Geometry check sheet. Reference: drawing and pictorial views, mm from the part's lowest x, y, z. Give positions to 0.01 mm unless a question says otherwise; leave off trailing zeros. Loops run counter-clockwise (first coordinate to the right, second up) from the corner with the lowest first, then second, coordinate; pieces in that order, holes last. Notation, with made-up numbers: (87, 42) - (110, 42) arc R14 ccw to (110, 60) - close; hole circle Ø10 at (19, 16.25). An arc over 180 degrees is marked (long way). Answer in a Markdown table with one row per item. Add a question column.
(1) Sectioned sample at D-D on z = 4.5. Enter the section's corners in (x, y), then the cut area to 3 significant figures.
(2) Sectioned sample at C-C on y = 15. Enter the section's corners in (x, z).
(3) Thickness scan on L1, parallel to X at y = 1.75, z = 5; L2, parallel to Z at x = 8, y = 17; L3, parallel to X at y = 7.75, z = 4.25. Record the ranges inside material, lowest first.
(4) Go/stop test with a flat-tipped pin: P1, Ø3, axis at x = 32, z = 6.5, coming from the -Y side. Record where the tip stops, or that it passes through.
(5) Sectioned sample at A-A on z = 6.5. Enter the section's corners in (x, y).
(6) Draft check along Z on the marked faces 1, 2, 3 and 4. Enter one of: released by +Z, released by -Z, zero draft, split by the parting line, or undercut.
(7) Sectioned sample at B-B on x = 32. Enter the section's corners in (y, z), then the cut area to 3 significant figures.
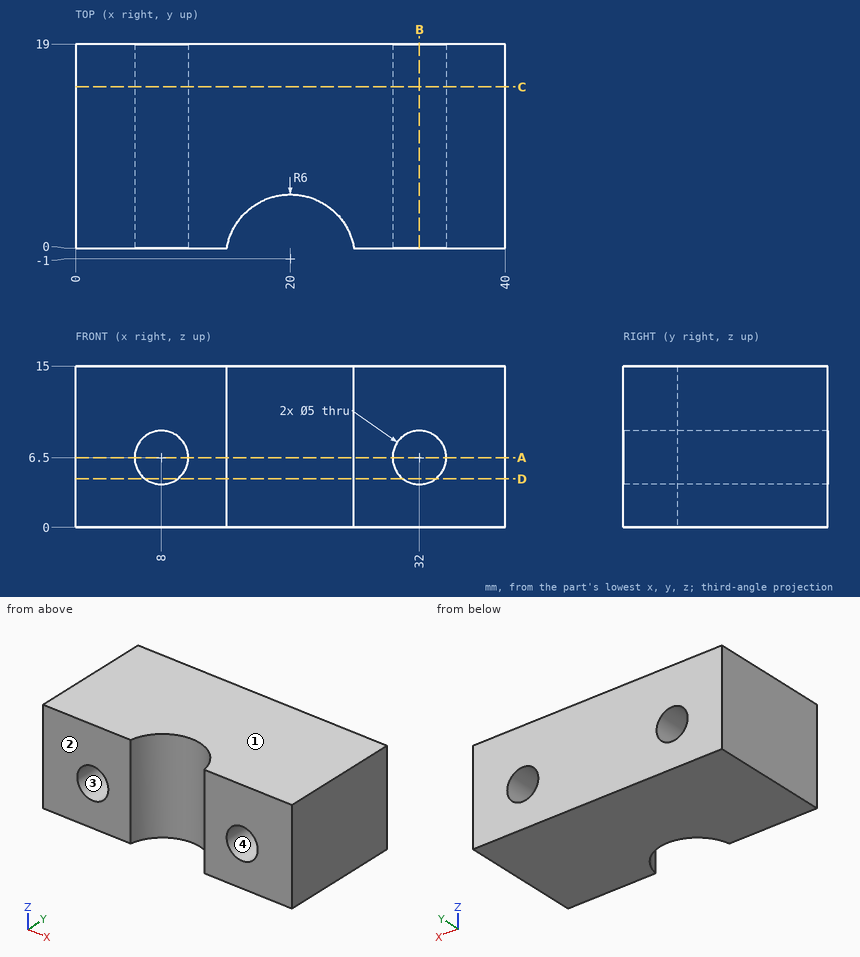
Reply:
| question | item | result |
|---|---|---|
| 1 | outline | (0, 0) - (6.5, 0) - (6.5, 19) - (0, 19) - close; (9.5, 0) - (14.08, 0) arc R6 cw to (25.92, 0) - (30.5, 0) - (30.5, 19) - (9.5, 19) - close; (33.5, 0) - (40, 0) - (40, 19) - (33.5, 19) - close |
| 1 | area | 601 mm^2 |
| 2 | outline | (0, 0) - (40, 0) - (40, 15) - (0, 15) - close; hole circle Ø5 at (8, 6.5); hole circle Ø5 at (32, 6.5) |
| 3 | L1 | 0 to 6, 10 to 14.67, 25.33 to 30, 34 to 40 |
| 3 | L2 | 0 to 4, 9 to 15 |
| 3 | L3 | 0 to 6.91, 9.09 to 30.91, 33.09 to 40 |
| 4 | P1 | through |
| 5 | outline | (0, 0) - (5.5, 0) - (5.5, 19) - (0, 19) - close; (10.5, 0) - (14.08, 0) arc R6 cw to (25.92, 0) - (29.5, 0) - (29.5, 19) - (10.5, 19) - close; (34.5, 0) - (40, 0) - (40, 19) - (34.5, 19) - close |
| 6 | face 1 | released by +Z |
| 6 | face 2 | zero draft |
| 6 | face 3 | undercut |
| 6 | face 4 | undercut |
| 7 | outline | (0, 0) - (19, 0) - (19, 4) - (0, 4) - close; (0, 9) - (19, 9) - (19, 15) - (0, 15) - close |
| 7 | area | 190 mm^2 |
